from build123d import *

# Parameters (mm, degrees)
SKETCH1_R                = 2.5000000000000036
BOSS_EXTRUDE1_DEPTH      = 20
BOSS_EXTRUDE3_START      = -30
BOSS_EXTRUDE3_DEPTH      = 30
FILLET1_R                = 2
FILLET1_OF_MIRROR2_R     = 2
BOSS_EXTRUDE5_DEPTH      = 5
BOSS_EXTRUDE5_DEPTH_BACK = 5
SKETCH10_W               = 5
SKETCH10_H               = 4.9999999999999964
SKETCH11_R               = 44.99999999999999
BOSS_EXTRUDE6_DEPTH      = 5
FILLET2_R                = 5


# Read off the part's stored shape, not the designer's step: Mirror3
with BuildPart() as part:
    # Sketch1 → Boss-Extrude1 (new body)
    with BuildSketch(Plane.XY):
        with BuildLine():
            Line((-3.7999999999999994, 5.999999999999999), (-3.799999999999992, -64.0238209295858))
            ThreePointArc((-3.800000000000015, -64.0238209295858), (-5.499999999999996, -67.99999999999999), (-3.8000000000000083, -71.97617907041419))
            Line((-3.799999999999991, -71.97617907041419), (-3.7999999999999896, -83.99999999999999))
            Line((-3.799999999999989, -83.99999999999999), (3.800000000000014, -83.99999999999999))
            Line((3.800000000000014, -83.99999999999999), (3.8000000000000123, -71.97617907041419))
            ThreePointArc((3.8000000000000083, -71.97617907041419), (5.499999999999996, -67.99999999999999), (3.800000000000015, -64.0238209295858))
            Line((3.800000000000011, -64.0238209295858), (3.7999999999999994, 6))
            ThreePointArc((3.800000000000001, 5.999999999999998), (0, 13.569343394379079), (-3.8000000000000016, 5.999999999999998))
        make_face()
        with Locations((0, -67.99999999999999)):
            Circle(SKETCH1_R, mode=Mode.SUBTRACT)
    extrude(amount=BOSS_EXTRUDE1_DEPTH)

    # Sketch5 → Boss-Extrude3 (add)
    with BuildSketch(Plane.XY.offset(BOSS_EXTRUDE3_START)):
        with BuildLine():
            ThreePointArc((4.738519293185978, 8.8308241011931), (-1.4911726556286193, 13.328597906421773), (-3.800000000000001, 5.999999999999998))
            Line((-3.8000000000000007, 5.999999999999998), (3.8000000000000007, 5.999999999999998))
            ThreePointArc((3.800000000000001, 5.999999999999999), (4.497773805228675, 7.339651445564482), (4.738519293185978, 8.830824101193098))
        make_face()
    boss_extrude3 = extrude(amount=BOSS_EXTRUDE3_DEPTH)

    # Fillet1
    fillet1_edges = [part.edges().sort_by_distance(p)[0] for p in [
        (0, 5.999999999999998, -30),
        (3.800000000000001, 5.999999999999998, -15),
        (4.44e-15, 13.569343394379077, -30),
        (-3.8000000000000016, 5.999999999999998, -15),
    ]]
    fillet(fillet1_edges, radius=FILLET1_R)

    # Mirror2: Boss-Extrude3 across plane
    add(boss_extrude3.mirror(Plane(origin=(0, 0, 10), x_dir=(1, 0, 0), z_dir=(0, 0, -1))))

    # Fillet1 of Mirror2
    fillet1_of_mirror2_edges = [part.edges().sort_by_distance(p)[0] for p in [
        (0, 5.999999999999998, 50),
        (3.800000000000001, 5.999999999999998, 35),
        (4.44e-15, 13.569343394379077, 50),
        (-3.8000000000000016, 5.999999999999998, 35),
    ]]
    fillet(fillet1_of_mirror2_edges, radius=FILLET1_OF_MIRROR2_R)

    # Mirror3: part across plane


with BuildPart() as part_1:
    add(part.part)
    add(part.part.mirror(Plane(origin=(0, -83.99999999999999, 20), x_dir=(0, 0, 1), z_dir=(0, -1, 0))))

    # Sketch10 → Boss-Extrude5 (add, two sides: drawn at the far end of the back side and taken through both)
    with BuildSketch(Plane(origin=(0, -83.99999999999999, 0), x_dir=(-1, 0, 0), z_dir=(0, -1, 0)).offset(-BOSS_EXTRUDE5_DEPTH_BACK)):
        Polygon((3.799999999999991, -20), (3.8000000000000007, 0), (78.79999999999998, 35.00000000000001), (78.79999999999998, 30.00000000000001), align=None)
        with Locations((81.29999999999998, 32.50000000000001)):
            Rectangle(SKETCH10_W, SKETCH10_H)
    extrude(amount=BOSS_EXTRUDE5_DEPTH + BOSS_EXTRUDE5_DEPTH_BACK)

    # Sketch11 → Boss-Extrude6 (add)
    with BuildSketch(Plane(origin=(0, 0, -35.00000000000001), x_dir=(-1, 0, 0), z_dir=(0, 0, -1))):
        with Locations((83.79999999999998, -83.99999999999999)):
            Circle(SKETCH11_R)
    extrude(amount=-BOSS_EXTRUDE6_DEPTH)

    # Fillet2
    fillet2_edges = [part_1.edges().sort_by_distance(p)[0] for p in [
        (-78.79999999999998, -83.99999999999999, -30.00000000000001),
        (-73.44285714285712, -88.99999999999999, -30.000000000000007),
        (-73.44285714285712, -78.99999999999999, -30.000000000000007),
    ]]
    fillet(fillet2_edges, radius=FILLET2_R)


solid = part_1.part
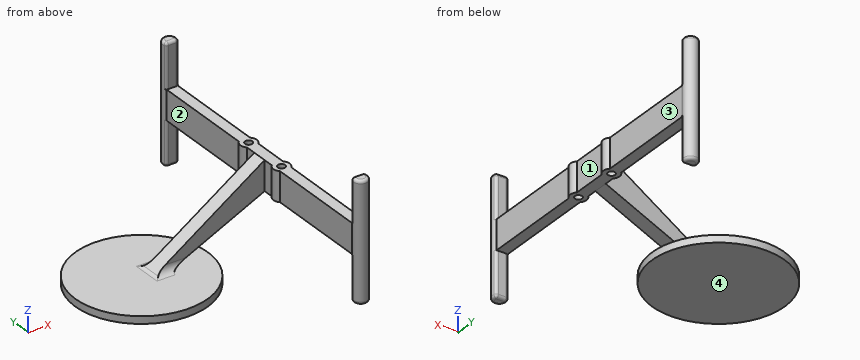
Model file for the job. Use its own axes, mm. Face numbers are marked on the shaded views. A direction names the side the tool comes from. Coordinates: 2 decimals unless noted, no trailing zeros. Order: outer loops, then holes, each group sorted by start corner. A loop starts at its lowest first (then second) coordinate and runs counter-clockwise, first axis right, second up. Notation, with made-up numbers: (-8, 37) -> (10, 37) arc R24 ccw to (10, 70) -> close; hole circle Ø6 at (31.5, 19.5). An arc over 180 degrees is marked (long way). Return JSON: item names as keys, results as strings. Group by question number.
Item 1: Saw through at B-B on x = -62.5. Write the cut outline in (y, z), then the cut area to 3 significant figures.
Item 2: Saw through at A-A on z = 7.5. Write the cut outline in (x, y).
Item 3: Saw through at D-D on z = 41.5. Write the cut outline in (x, y).
Item 4: Wall check: line 1 along Z through (x, y) = (-55.5, -57); line 2 along Z through (x, y) = (-3, -166); line 3 along X through (y, z) = (-80, -16). Give the ranges that are in metal, low to high. Write a range as [from, to].
Item 5: Pull direction Y, two halves, no side cores. Call the marked faces 3 and 4: pulls with the +Y half, pulls with the -Y half, needs draft (parallel to the pull), parting line crosses it, or undercut.
Item 6: Saw through at C-C on y = -100. Write the cut outline in (x, z).
Item 7: Tool access for the marked faces 1 and 2: list every direction of +Z, -Z, +X, -X, +Y, -Y with a clear straight run to the whole face (end or side of a thin tool).
Item 8: Flat gauge pins, fed straight in: P1, Ø10, axis at y = -133.5, z = 10.5, coming from the +X side; P2, Ø12, axis at x = 2, y = -74, coming from the -Z side; P3, Ø22.5, axis at x = -50, z = -2, coming from the -Y side; P4, Ø3, axis at x = 0, y = -68, coming from the +Z side. Where does each tip first touch, or does it go through?
Values found:
{
 "1": {"outline": "(-123.64, -35) -> (-44.36, -35) -> (-44.36, -30) -> (-123.64, -30) -> close; (-89.61, -27.39) -> (-78.39, -27.39) arc R5 cw to (-79, -25) -> (-79, -19.13) -> (-89, -19.13) -> (-89, -25) arc R5 cw to start", "area": "480 mm2"},
 "2": {"outline": "(-22.55, -89) -> (-3.8, -89) -> (-3.8, -96.02) arc R5.5 ccw to (-3.8, -103.98) -> (-3.8, -174) arc R4.74 ccw (long way) to (3.8, -174) -> (3.8, -103.98) arc R5.5 ccw to (3.8, -96.02) -> (3.8, -71.98) arc R5.5 ccw to (3.8, -64.02) -> (3.8, 6) arc R4.74 ccw (long way) to (-3.8, 6) -> (-3.8, -64.02) arc R5.5 ccw to (-3.8, -71.98) -> (-3.8, -79) -> (-22.55, -79) -> close; hole circle Ø5 at (0, -100); hole circle Ø5 at (0, -68)"},
 "3": {"outline": "(-4.52, -175.39) arc R4.74 ccw (long way) to (4.52, -175.39) arc R2 ccw to (2.61, -174) -> (-2.61, -174) arc R2 ccw to start; (-4.52, 7.39) arc R2 ccw to (-2.61, 6) -> (2.61, 6) arc R2 ccw to (4.52, 7.39) arc R4.74 ccw (long way) to start"},
 "4": {"line 1": "z = [-35, -30]", "line 2": "z = [0, 20]", "line 3": "x = [-57.8, -38.09]"},
 "5": {"face 3": "undercut", "face 4": "needs draft"},
 "6": {"outline": "(-125.86, -35) -> (-41.74, -35) -> (-41.74, -30) -> (-125.86, -30) -> close; (-5.5, 0) -> (-2.5, 0) -> (-2.5, 20) -> (-5.5, 20) -> close; (2.5, 0) -> (5.5, 0) -> (5.5, 20) -> (2.5, 20) -> close"},
 "7": {"face 1": "+Z, -Z, +X", "face 2": "+Z, -Z, -X"},
 "8": {"P1": "stops at x = 3.8", "P2": "stops at z = 0", "P3": "stops at y = -89", "P4": "passes through"}
}
